```python
from build123d import *

# Parameters (mm, degrees)
EXTRUDE1_DEPTH = 5.953125
SKETCH2_W      = 2.413
SKETCH2_H      = 5.953125


with BuildPart() as part:
    # Sketch1 → Extrude1 (new body)
    with BuildSketch(Plane(origin=(0, 0, 0), x_dir=(1, 0, 0), z_dir=(0, 1, 0))):
        Polygon((0, 5.499261314), (-4.7625, 2.749630657), (-4.7625, -2.749630657), (0, -5.499261314), (4.7625, -2.749630657), (4.7625, 2.749630657), align=None)
    extrude(amount=EXTRUDE1_DEPTH)


with BuildPart() as body_2:
    # Sketch2 → Revolve1 (revolve)
    with BuildSketch(Plane(origin=(0, 0, 0), x_dir=(0, 0, -1), z_dir=(1, 0, 0))):
        with Locations((1.2065, 2.9765625)):
            Rectangle(SKETCH2_W, SKETCH2_H)
    revolve(axis=Axis((0, -2.413, 0), (0, 1, 0)))


with BuildPart() as part_1:
    add(part.part)

    # Combine1: cut body 2
    add(body_2.part, mode=Mode.SUBTRACT)

    # Sketch5 → Cut-Revolve3 (revolve, cut)
    with BuildSketch(Plane(origin=(0, 0, 0), x_dir=(0, 0, -1), z_dir=(1, 0, 0))):
        with BuildLine():
            Line((0, 0), (4.7625, 0))
            Line((4.7625, 0), (5.499261314, 0.343557443))
            Line((5.499261314, 0.343557443), (5.499261314, 4.617380057))
            Line((5.499261314, 4.617380057), (4.7625, 4.9609375))
            ThreePointArc((4.7625, 4.9609375), (4.471895009, 5.662520009), (3.7703125, 5.953125))
            Line((3.7703125, 5.953125), (3.7703125, 7.223125))
            Line((3.7703125, 7.223125), (6.769261314, 7.223125))
            Line((6.769261314, 7.223125), (6.769261314, -1.27))
            Line((6.769261314, -1.27), (0, -1.27))
            Line((0, -1.27), (0, 0))
        make_face()
    revolve(axis=Axis((0, 0, 0), (0, 1, 0)), mode=Mode.SUBTRACT)


solid = part_1.part
```
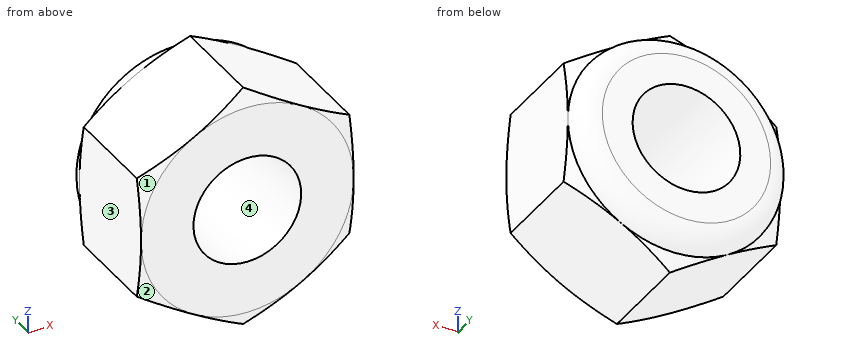
Here's how the part is built. I have some questions about the finished solid (model axes, mm). Face numbers are marked on the shaded views. Give positions to 0.01 mm unless a question says otherwise; leave off trailing zeros. Loops run counter-clockwise (first coordinate to the right, second up) from the corner with the lowest first, then second, coordinate; pieces in that order, holes last. Notation, with made-up numbers: (10, -38) -> (53, -38) arc R31 ccw to (53, -10) -> close; hole circle Ø10 at (15, -0.75). An arc over 180 degrees is marked (long way). Use one line per item in the form item = value. Start each with the question number.
1) Imagine slicing it at A-A (y = 0.9). Please give me the cut outline in (x, z).
2) For P1, Ø1.5, axis at y = 2, z = -4, coming from the -X side, with a flat end and sliding along its axis, tell me the tip position at first contact or that it passes through.
3) Thinking about a two-plate mould opening in Z: for the marked faces 1, 2, 3 and 4, which applies, +Z half, -Z half, draft (parallel to the pull), parting line (faces both ways), or undercut?
4) Please list where these lines run through material, in increasing order: line 1 along X through (y, z) = (2.5, 0); line 2 along Z through (x, y) = (-3, 2.4); line 3 along X through (y, z) = (5.15, -1.75).
Check values:
q1.outline = (-4.76, -2.75) -> (0, -5.5) -> (4.76, -2.75) -> (4.76, 2.75) -> (0, 5.5) -> (-4.76, 2.75) -> close; hole circle Ø4.83 at (0, 0)
q2.P1 = -3.9
q3.face_1 = +Z half
q3.face_2 = -Z half
q3.face_3 = draft
q3.face_4 = undercut
q4.line_1 = -4.76 to -2.41, 2.41 to 4.76
q4.line_2 = -3.77 to 3.77
q4.line_3 = -4.41 to -1.66, 1.66 to 4.41
